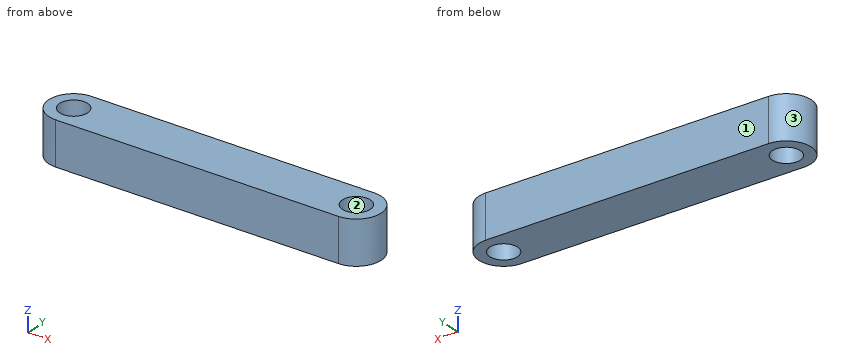
Autodesk Inventor part; units mm, degrees
ref_plane "YZ Plane" through (0, 0, 0) normal (1, 0, 0) x (0, 1, 0)
ref_plane "XZ Plane" through (0, 0, 0) normal (0, 1, 0) x (-1, 0, 0)
ref_plane "XY Plane" through (0, 0, 0) normal (0, 0, 1) x (1, 0, 0)
sketch "Sketch1" plane through (0, 0, 0) normal (0, 0, 1) x (1, 0, 0)
  circle A0 centre (-22.75, 0) radius 2.25
  circle A1 centre (22.75, 0) radius 2.25
  line L0 (-22.75, 0) -> (22.75, 0) construction
  line L1 (-22.75, -4) -> (22.75, -4)
  line L2 (22.75, 4) -> (-22.75, 4)
  arc A2 (-22.75, 4) -> (-22.75, -4) centre (-22.75, 0) ccw
  arc A3 (22.75, -4) -> (22.75, 4) centre (22.75, 0) ccw
  point P0 (0, 0)
  point P1 (0, 0)
  dimension "d0" = 8
extrude "Extrusion1" add sketch "Sketch1" along normal blind 7
scale "Scale1" factors (0.5, 0.5, 0.5) then translate (0, -2, 3.5) bodies 1
properties part number "MassiveToe1"
Geometry check sheet. Reference: the model listing, model coordinates, mm. Face numbers are marked on the shaded views. Round coordinates to 2 decimals unless told otherwise and drop trailing zeros. Loops run counter-clockwise (first coordinate to the right, second up) from the corner with the lowest first, then second, coordinate; pieces in that order, holes last. Notation, with made-up numbers: (56.5, 47) - (84.5, 47) arc R26 cw to (84.5, 65) - close; hole circle Ø11 at (27.25, 61.25). An arc over 180 degrees is marked (long way). Answer as CSV lines item,"result".
(1) Cross-section at A-A, the plane y = -2. Enter the section's corners in (x, z) (3 decimals), and give its area (3 significant figures).
Output values:
outline,"(-13.375, 3.5) - (-12.5, 3.5) - (-12.5, 7) - (-13.375, 7) - close; (-10.25, 3.5) - (10.25, 3.5) - (10.25, 7) - (-10.25, 7) - close; (12.5, 3.5) - (13.375, 3.5) - (13.375, 7) - (12.5, 7) - close"
area,"77.9 mm²"
(2) Release check for a two-part mould opening along Y. For the marked faces 1, 2 and 3 record: released by +Y, released by -Y, zero draft, split by the parting line, or undercut.
Output values:
face 1,"released by +Y"
face 2,"undercut"
face 3,"split by the parting line"
(3) Material ranges on line 1 along X through (y, z) = (-2.9, 4.8); line 2 along X through (y, z) = (-1.65, 5.95); line 3 along Y through (x, z) = (-12, 4.75), recorded low to high.
Output values:
line 1,"x = -13.16 to -12.05, -10.7 to 10.7, 12.05 to 13.16"
line 2,"x = -13.34 to -12.44, -10.31 to 10.31, 12.44 to 13.34"
line 3,"y = -3.9 to -2.94, -1.06 to -0.1"
(4) Cross-section at B-B, the plane z = 5.8. Enter the section's corners in (x, y) (3 decimals), and give its area (3 significant figures).
Output values:
outline,"(-11.375, -4) - (11.375, -4) arc R2 ccw to (11.375, 0) - (-11.375, 0) arc R2 ccw to start; hole circle Ø2.25 at (-11.375, -2); hole circle Ø2.25 at (11.375, -2)"
area,"95.6 mm²"
(5) Cross-section at C-C, the plane x = -11. Enter the section's corners in (y, z).
Output values:
outline,"(-4, 3.5) - (-3.06, 3.5) - (-3.06, 7) - (-4, 7) - close; (-0.94, 3.5) - (0, 3.5) - (0, 7) - (-0.94, 7) - close"
(6) Depth check by flat-ended pin: pin 1 Ø1 at (y, z) = (-1.5, 6) entering from -X (3 decimals). Enter the tip coordinate at first touch or a pass-through.
Output values:
pin 1,"stops at x = -13.375"
(7) Cross-section at D-D, the plane y = -0.35. Enter the section's corners in (x, z).
Output values:
outline,"(-12.51, 3.5) - (12.51, 3.5) - (12.51, 7) - (-12.51, 7) - close"
